Can you work these out from the model? Positions are in its coordinate system, mm. Face numbers are marked on the shaded views. A direction names the side the tool comes from. Coordinates: 2 decimals unless noted, no trailing zeros. Order: outer loops, then holes, each group sorted by start corner. A loop starts at its lowest first (then second) coordinate and runs counter-clockwise, first axis right, second up.
```python
from build123d import *

# Parameters (mm, degrees)
F0_W      = 143
F0_H      = 84
F1_DEPTH  = 1.5
F2_R      = 2
F3_DEPTH  = 12.5
F4_W      = 10.44
F4_H      = 10.76
F5_DEPTH  = 18.62
F6_W      = 7.8
F6_H      = 30
F7_DEPTH  = 10.3
F8_W      = 8.7
F8_H      = 20.25
F9_DEPTH  = 9
F10_W     = 110
F10_H     = 15.2
F11_DEPTH = 19
F12_W     = 12.3
F12_H     = 16.3
F13_DEPTH = 11


with BuildPart() as f1:
    # F0 (on Top) → F1 (new body)
    with BuildSketch(Plane.XY):
        with Locations((71.5, 42)):
            Rectangle(F0_W, F0_H)
    extrude(amount=F1_DEPTH)

    # F2 (on face) → F3 (cut, symmetric)
    with BuildSketch(Plane.XY.offset(1.5)):
        with Locations((139, 4)):
            Circle(F2_R)
        with Locations((139, 80)):
            Circle(F2_R)
        with Locations((4, 80)):
            Circle(F2_R)
        with Locations((4, 4)):
            Circle(F2_R)
    extrude(amount=F3_DEPTH, both=True, mode=Mode.SUBTRACT)

    # F4 (on face) → F5 (join)
    with BuildSketch(Plane.XY.offset(1.5)):
        with Locations((136.58, 68.62)):
            Rectangle(F4_W, F4_H)
        with Locations((136.58, 42.36)):
            Rectangle(F4_W, F4_H)
    extrude(amount=F5_DEPTH)

    # F6 (on face) → F7 (join)
    with BuildSketch(Plane.XY.offset(1.5)):
        with Locations((135.4, 22.13)):
            Rectangle(F6_W, F6_H)
    extrude(amount=F7_DEPTH)

    # F8 (on face) → F9 (join)
    with BuildSketch(Plane.XY.offset(1.5)):
        with Locations((5.85, 64.305)):
            Rectangle(F8_W, F8_H)
        with Locations((5.85, 42.555)):
            Rectangle(F8_W, F8_H)
    extrude(amount=F9_DEPTH)

    # F10 (on face) → F11 (join)
    with BuildSketch(Plane.XY.offset(1.5)):
        with Locations((58.7, 16.4)):
            Rectangle(F10_W, F10_H)
    extrude(amount=F11_DEPTH)

    # F12 (on face) → F13 (join)
    with BuildSketch(Plane.XY.offset(1.5)):
        with Locations((115.35, 75.85)):
            Rectangle(F12_W, F12_H)
    extrude(amount=F13_DEPTH)


solid = f1.part
```
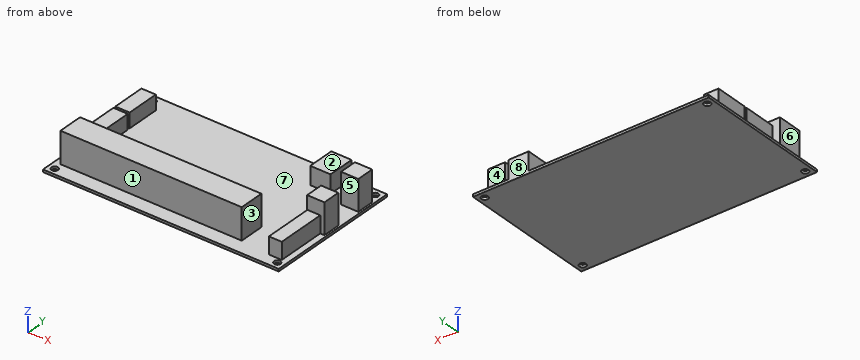
1. On a 3-axis mill with a long thin cutter (end or side, diameter ignored), from which of +Z, -Z, +X, -X, +Y, -Y can I reach the whole of each face in a straight line? I mean the marked faces 1, 2, 3, 4 and 5. Say none if no direction works.
Completed:
face 1: +Z, -X, -Y
face 2: +Z, -X, +Y
face 3: +Z, -Y
face 4: +Z, +X, +Y
face 5: +Z, +X
2. Imagine slicing it at B-B on y = 4. Please give me the cut outline in (x, z).
Completed:
outline: (0, 0) - (2, 0) - (2, 1.5) - (0, 1.5) - close; (6, 0) - (137, 0) - (137, 1.5) - (6, 1.5) - close; (141, 0) - (143, 0) - (143, 1.5) - (141, 1.5) - close
3. Please list where these lines run through material, in increasing order: probe 1 along Y at (x, z) = (4, 0.75); probe 2 along Y at (x, z) = (7.5, 8.25); probe 3 along X at (y, z) = (16, 8.75).
Completed:
probe 1: y = 0 to 2, 6 to 78, 82 to 84
probe 2: y = 8.8 to 24, 32.43 to 52.68, 54.18 to 74.43
probe 3: x = 3.7 to 113.7, 131.5 to 139.3
4. Imagine slicing it at C-C on z = 16. Please give me the cut outline in (x, y).
Completed:
outline: (3.7, 8.8) - (113.7, 8.8) - (113.7, 24) - (3.7, 24) - close; (131.36, 36.98) - (141.8, 36.98) - (141.8, 47.74) - (131.36, 47.74) - close; (131.36, 63.24) - (141.8, 63.24) - (141.8, 74) - (131.36, 74) - close
5. Imagine slicing it at D-D on y = 59. Please give me the cut outline in (x, z), then the cut area to 3 significant figures.
Completed:
outline: (0, 0) - (143, 0) - (143, 1.5) - (10.2, 1.5) - (10.2, 10.5) - (1.5, 10.5) - (1.5, 1.5) - (0, 1.5) - close
area: 293 mm2
6. I'm going to push flat-ended pins straight in: pin 1 (2.5 mm diameter, centred on y = 46, z = 7, fed in from -X); pin 2 (6 mm diameter, centred on x = 27.5, z = 11.5, fed in from -Y); pin 3 (2.5 mm diameter, centred on x = 5, z = 4, fed in from +Y). Where does each tip first touch, or does it pass through?
Completed:
pin 1: stops at x = 1.5
pin 2: stops at y = 8.8
pin 3: stops at y = 74.43
7. Thinking about a two-plate mould opening in X: for the marked faces 6, 7 and 8, which applies, pulls with the +X half, pulls with the -X half, needs draft (parallel to the pull), parting line crosses it, or undercut?
Completed:
face 6: pulls with the -X half
face 7: undercut
face 8: needs draft
8. Imagine slicing it at A-A on z = 6.5. Please give me the cut outline in (x, y).
Completed:
outline: (1.5, 32.43) - (10.2, 32.43) - (10.2, 52.68) - (1.5, 52.68) - close; (1.5, 54.18) - (10.2, 54.18) - (10.2, 74.43) - (1.5, 74.43) - close; (3.7, 8.8) - (113.7, 8.8) - (113.7, 24) - (3.7, 24) - close; (109.2, 67.7) - (121.5, 67.7) - (121.5, 84) - (109.2, 84) - close; (131.36, 36.98) - (131.5, 36.98) - (131.5, 7.13) - (139.3, 7.13) - (139.3, 36.98) - (141.8, 36.98) - (141.8, 47.74) - (131.36, 47.74) - close; (131.36, 63.24) - (141.8, 63.24) - (141.8, 74) - (131.36, 74) - close
